Job drawing, mm, ordinate dimensions from the low corner. One solid piece. Round coordinates to 2 decimals unless told otherwise and drop trailing zeros. Write each loop counter-clockwise with the first axis right and the second up, starting at its lowest first coordinate (ties: lowest second). Pieces come first, ordered by that corner, then holes. Notation, with made-up numbers: M -23,-30.5 L 14,-30.5 A26 cw 14,-7.5 Z; hole C 75,-38.5 d8. An arc over 180 degrees is marked long. Answer as a JSON object with one key per item and string values. Group by question number.
1. Band-saw the part on D-D, the plane y = 127.5. Write the cut outline in (x, z), plus the area to 3 significant figures.
2. Band-saw the part on A-A, the plane z = 1.5. Write the cut outline in (x, y), plus the area to 3 significant figures.
3. Band-saw the part on C-C, the plane z = 18. Write the cut outline in (x, y).
4. Band-saw the part on B-B, the plane x = 0.8. Write the cut outline in (y, z), plus the area to 3 significant figures.
5. Drop flat-ended pins along their axis: pin 1 (0.9 mm diameter, centred on x = 2, z = 6.5, fed in from +Y); pin 2 (0.9 mm diameter, centred on x = 1.5, z = 7, fed in from -Y); pin 3 (2 mm diameter, centred on y = 109, z = 5.5, fed in from -X); pin 4 (1.5 mm diameter, centred on x = 1.5, y = 36.5, fed in from -Z). Give the stop position or say it passes through.
6. Drill centre lines: line 1 (Y direction, x = 2.65, z = 8.75); line 2 (Y direction, x = 2.55, z = 1.5); line 3 (Z direction, x = 1.05, y = 129.5). Where is each one in solid material? Low to high. Write a range as from..to.
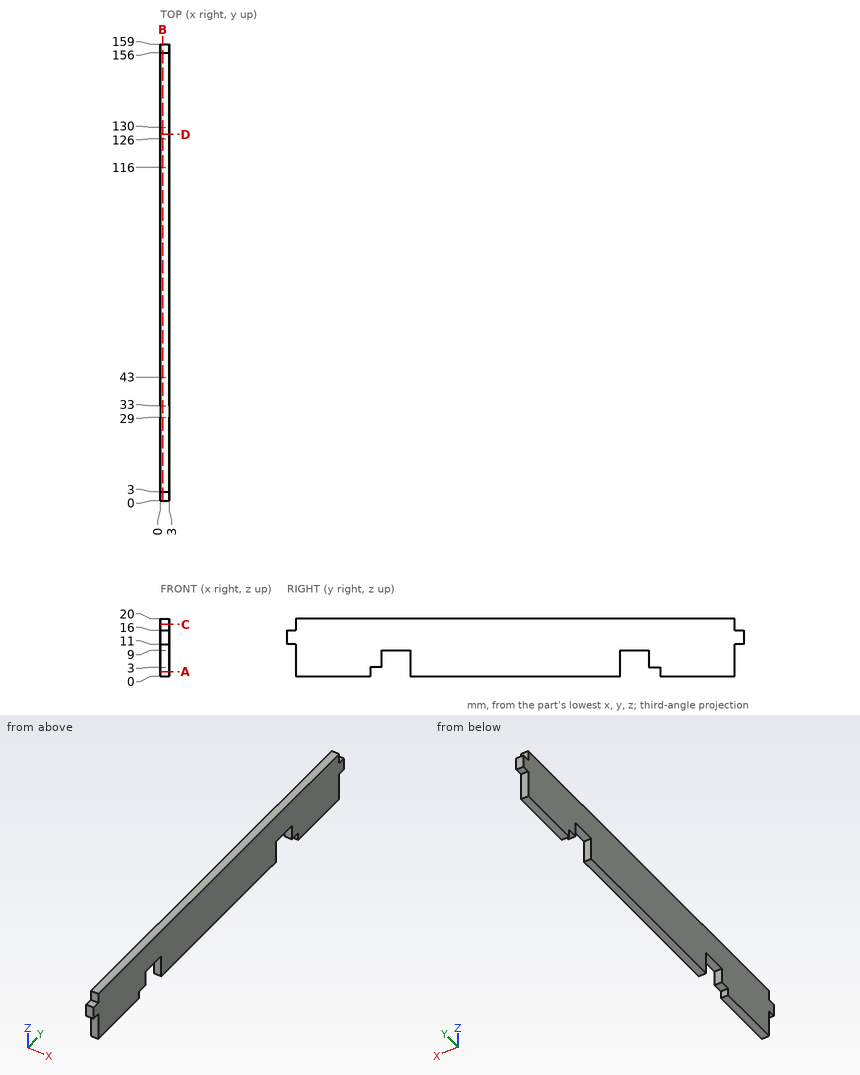
Worked answers:
{
 "1": {"outline": "M 0,3 L 3,3 L 3,20 L 0,20 Z", "area": "51.0 mm^2"},
 "2": {"outline": "M 0,3 L 3,3 L 3,29 L 0,29 Z; M 0,43 L 3,43 L 3,116 L 0,116 Z; M 0,130 L 3,130 L 3,156 L 0,156 Z", "area": "375 mm^2"},
 "3": {"outline": "M 0,3 L 3,3 L 3,156 L 0,156 Z"},
 "4": {"outline": "M 0,11 L 3,11 L 3,0 L 29,0 L 29,3 L 33,3 L 33,9 L 43,9 L 43,0 L 116,0 L 116,9 L 126,9 L 126,3 L 130,3 L 130,0 L 156,0 L 156,11 L 159,11 L 159,16 L 156,16 L 156,20 L 3,20 L 3,16 L 0,16 Z", "area": "2,890 mm^2"},
 "5": {"pin 1": "stops at y = 156", "pin 2": "stops at y = 3", "pin 3": "stops at x = 0", "pin 4": "stops at z = 9"},
 "6": {"line 1": "y = 3..33, 43..116, 126..156", "line 2": "y = 3..29, 43..116, 130..156", "line 3": "z = 3..20"}
}
